Design review of the part built by this model. Coordinates are the model's own, in mm. A direction names the side the tool comes from. Round coordinates to 2 decimals unless told otherwise and drop trailing zeros. Use CSV: the item, a comma, the result in double quotes. Start each with the question number.
Autodesk Inventor part; units mm, degrees
ref_plane "YZ Plane" through (0, 0, 0) normal (1, 0, 0) x (0, 1, 0)
ref_plane "XZ Plane" through (0, 0, 0) normal (0, 1, 0) x (-1, 0, 0)
ref_plane "XY Plane" through (0, 0, 0) normal (0, 0, 1) x (1, 0, 0)
sketch "Sketch1" plane through (0, 0, 0) normal (0, 0, 1) x (1, 0, 0)
  circle A0 centre (0, 0) radius 20.6375
  circle A1 centre (0, 0) radius 17.4625
  dimension "d0" = 41.275
  dimension "d1" = 34.925
extrude "Extrusion1" add sketch "Sketch1" along normal blind 1.5875
sketch "Sketch2" plane through (0, 0, 1.5875) normal (0, 0, 1) x (1, 0, 0)
  circle A0 centre (0, 0) radius 17.4625
  circle A1 centre (0, 0) radius 20.6375
  circle A2 centre (0, 0) radius 19.05
  dimension "d4" = 38.1
extrude "Extrusion2" add sketch "Sketch2" along normal blind 1.5875 contours A2
sketch "Sketch3" plane through (0, 0, 3.175) normal (0, 0, 1) x (1, 0, 0)
  circle A0 centre (0, 0) radius 19.05
  circle A1 centre (0, 0) radius 22.225
  dimension "d7" = 44.45
extrude "Extrusion3" add sketch "Sketch3" along normal blind 1.5875 contours A0 | A1
chamfer "Chamfer1" distance 4.7625 distance2 1.5875 1 edges at (-22.225, 0, 4.7625) measured on face at (2.0252, -4.4852, 4.7625)
chamfer "Chamfer2" distance 1.5875 angle 45 1 edges at (-17.4625, 0, 0)
properties part number "Plastic Plug" material "Plastic, Opaque Black"
Q1. Tool access review of faces 4 (the flat face through (0, 0, 4.762)), 5 (the cylindrical face through (-4.474, 20.147, 0.783)), 6 (the cylindrical face through (-15.12, 11.59, 2.37)): name each direction out of +Z, -Z, +X, -X, +Y, -Y from which nothing blocks a thin tool from reaching the whole face with its end or side.
Q2. The part is to be moulded in two halves that separate along X. For faces 1 (the conical face through (-3.85, 17.339, 4.663)), 2 (the cylindrical face through (-13.858, 10.626, 2.37)), 3 (the flat face through (6.02, -18.25, 1.588)), say which applies: +X half, -X half, draft (parallel to the pull), parting line (faces both ways), or undercut.
Q3. For L1, parallel to Y at x = 0, z = 2.7; L2, parallel to Z at x = 3, y = 0.5 (1 decimal); L3, parallel to X at y = -3.5, z = 2.4, list the stretches that pass through material, from the lowest coordinate up. Write a range as [from, to].
Q4. Clearance check with flat-ended pins moving along their axes: pin 1 (1.5 mm diameter, centred on x = -13, z = 0.5, fed in from +Y); pin 2 (1.5 mm diameter, centred on x = -8, y = 0, fed in from -Z) (3 decimals); pin 3 (1.5 mm diameter, centred on x = -15.5, y = -7.5, fed in from -Z). State where each tip first meets the part, or that it passes through.
Findings below:
1,face 4,"+Z, +X, -X, +Y, -Y"
1,face 5,"-Z"
1,face 6,"none"
2,face 1,"parting line"
2,face 2,"undercut"
2,face 3,"draft"
3,L1,"y = [-19.05, -17.46], [17.46, 19.05]"
3,L2,"z = [3.2, 4.8]"
3,L3,"x = [-18.73, -17.11], [17.11, 18.73]"
4,pin 1,"stops at y = 16.61"
4,pin 2,"stops at z = 3.175"
4,pin 3,"stops at z = 1.08"
